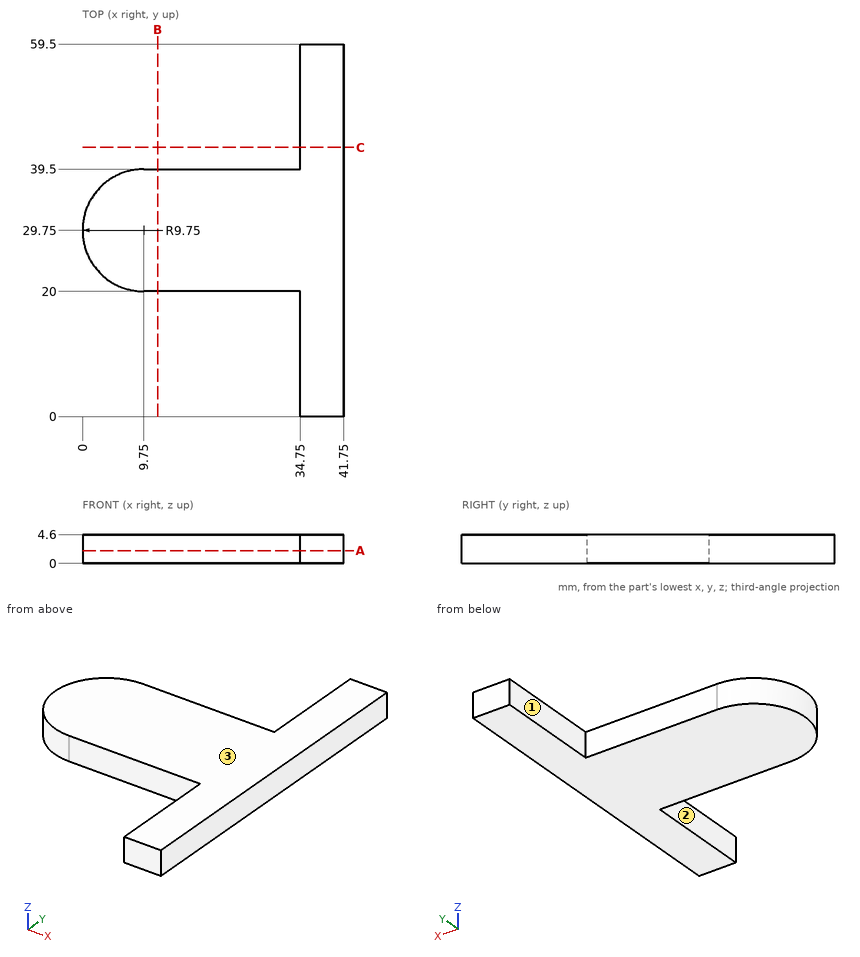
Source: three-view drawing plus pictorial views. Frame: mm from the lowest corner of the part. A direction names the side the tool comes from. Round coordinates to 2 decimals unless told otherwise and drop trailing zeros. Order: outer loops, then holes, each group sorted by start corner. A loop starts at its lowest first (then second) coordinate and runs counter-clockwise, first axis right, second up. Notation, with made-up numbers: (-8, 81.25) - (44, 81.25) arc R10 ccw to (44, 94.25) - close; hole circle Ø9 at (58, 64.5). An arc over 180 degrees is marked (long way). Answer in a Markdown table with one row per item.
Item 1: Pin query (flat end, axial travel): pin 1 (1.4 mm diameter, centred on y = 47, z = 2, fed in from -X); pin 2 (1.4 mm diameter, centred on x = 17, z = 2.5, fed in from -Y); pin 3 (2 mm diameter, centred on x = 17.5, z = 3, fed in from +Y). Return the tip coordinate at first contact, or that it passes through.
Model answer:
| item | result |
|---|---|
| pin 1 | stops at x = 34.75 |
| pin 2 | stops at y = 20 |
| pin 3 | stops at y = 39.5 |
Item 2: Section query A-A (z = 2.05). Return the cut outline in (x, y), then the cut area to 3 significant figures.
Model answer:
| item | result |
|---|---|
| outline | (9.75, 20) - (34.75, 20) - (34.75, 0) - (41.75, 0) - (41.75, 59.5) - (34.75, 59.5) - (34.75, 39.5) - (9.75, 39.5) arc R9.75 ccw to start |
| area | 1,050 mm² |
Item 3: Reachability of the marked faces 1, 2 and 3 from +Z, -Z, +X, -X, +Y, -Y: full face, straight path, thin tool, end or side. Return the list, or none.
Model answer:
| item | result |
|---|---|
| face 1 | +Z, -Z, -X, +Y |
| face 2 | +Z, -Z, -X, -Y |
| face 3 | +Z, +X, -X, +Y, -Y |
Item 4: Section query C-C (y = 43). Return the cut outline in (x, z), then the cut area to 3 significant figures.
Model answer:
| item | result |
|---|---|
| outline | (34.75, 0) - (41.75, 0) - (41.75, 4.6) - (34.75, 4.6) - close |
| area | 32.2 mm² |
Item 5: Line query: line 1 (Y direction, x = 9.5, z = 4.25); line 2 (X direction, y = 41, z = 1); line 3 (Y direction, x = 4.5, z = 4.2). Output: solid intervals per line, ascending.
Model answer:
| item | result |
|---|---|
| line 1 | y = 20 to 39.5 |
| line 2 | x = 34.75 to 41.75 |
| line 3 | y = 21.53 to 37.97 |
Item 6: Section query B-B (x = 12). Return the cut outline in (y, z).
Model answer:
| item | result |
|---|---|
| outline | (20, 0) - (39.5, 0) - (39.5, 4.6) - (20, 4.6) - close |
